Geometry check sheet. Reference: the model listing, model coordinates, mm. A direction names the side the tool comes from. Round coordinates to 2 decimals unless told otherwise and drop trailing zeros. Write each loop counter-clockwise with the first axis right and the second up, starting at its lowest first coordinate (ties: lowest second). Pieces come first, ordered by that corner, then holes. Notation, with made-up numbers: M 68,-28.75 L 73,-28.75 A20 cw 73,-20.75 Z; hole C 77,26.25 d4. An arc over 180 degrees is marked long. Answer in a Markdown table with one row per item. Add a question column.
Autodesk Inventor part; units mm, degrees
ref_plane "YZ Plane" through (0, 0, 0) normal (1, 0, 0) x (0, 1, 0)
ref_plane "XZ Plane" through (0, 0, 0) normal (0, 1, 0) x (-1, 0, 0)
ref_plane "XY Plane" through (0, 0, 0) normal (0, 0, 1) x (1, 0, 0)
sketch "Эскиз1" plane through (0, 0, 0) normal (0, 0, 1) x (1, 0, 0)
  line L0 (115, 5) -> (-115, 5)
  line L1 (-115, 5) -> (-115, -5)
  line L2 (-115, -5) -> (115, -5)
  line L3 (115, -5) -> (115, 5)
  line L4 (115, 5) -> (-115, -5) construction
  line L5 (-115, 5) -> (115, -5) construction
  arc A0 (0, 0) -> (-115, -5) centre (-47.7882, -225.8713) ccw
  arc A1 (115, -5) -> (0, 0) centre (47.7882, -225.8713) ccw
  line L6 (115, 10) -> (-115, 10)
  line L7 (-115, 10) -> (-115, 0)
  line L8 (-115, 0) -> (115, 0)
  line L9 (115, 0) -> (115, 10)
  line L10 (115, 10) -> (-115, 0) construction
  line L11 (-115, 10) -> (115, 0) construction
  arc A2 (0, 5) -> (-115, 0) centre (-47.7882, -220.8713) ccw
  arc A3 (115, 0) -> (0, 5) centre (47.7882, -220.8713) ccw
  line L12 (-115, -5) -> (-95.5764, 5)
  line L13 (115, -5) -> (95.5764, 5)
  line L14 (1.5, 15) -> (-1.5, 15)
  line L15 (-1.5, 15) -> (-1.5, -5)
  line L16 (-1.5, -5) -> (1.5, -5)
  line L17 (1.5, -5) -> (1.5, 15)
  line L18 (1.5, 15) -> (-1.5, -5) construction
  line L19 (-1.5, 15) -> (1.5, -5) construction
  line L20 (-1.5, 5) -> (1.5, 5)
  line L21 (1.5, 5) -> (1.5, 20)
  line L22 (1.5, 20) -> (-1.5, 20)
  line L23 (-1.5, 20) -> (-1.5, 5)
  circle A4 centre (0, 15) radius 1.5
  line L24 (1.5, 20) -> (4.5, 20)
  line L25 (4.5, 20) -> (4.5, 5)
  line L26 (4.5, 5) -> (1.5, 5)
  line L27 (1.5, 5) -> (1.5, 20)
  line L28 (-1.5, 20) -> (-4.5, 20)
  line L29 (-4.5, 20) -> (-4.5, 5)
  line L30 (-4.5, 5) -> (-1.5, 5)
  line L31 (-1.5, 5) -> (-1.5, 20)
  line L32 (-47.7882, 10) -> (-4.5, 10)
  line L33 (4.5, 10) -> (47.7882, 10)
  line L34 (4.5, 13.5) -> (-4.5, 13.5)
  line L35 (-4.5, 13.5) -> (-4.5, 16.5)
  line L36 (-4.5, 16.5) -> (4.5, 16.5)
  line L37 (4.5, 16.5) -> (4.5, 13.5)
  line L38 (4.5, 13.5) -> (-4.5, 16.5) construction
  line L39 (-4.5, 13.5) -> (4.5, 16.5) construction
  line L40 (4.5, 12.5) -> (-4.5, 12.5)
  line L41 (-4.5, 12.5) -> (-4.5, 17.5)
  line L42 (-4.5, 17.5) -> (4.5, 17.5)
  line L43 (4.5, 17.5) -> (4.5, 12.5)
  line L44 (4.5, 12.5) -> (-4.5, 17.5) construction
  line L45 (-4.5, 12.5) -> (4.5, 17.5) construction
  point P0 (1.5, 5.3122)
  point P1 (4.5, 5.9054)
  point P2 (-4.5, 5.9054)
  point P3 (-1.5, 5.3122)
  dimension "d6" = 3
  dimension "d0" = 230
  dimension "d1" = 10
  dimension "d4" = 3
  dimension "d5" = 15
  dimension "d7" = 3
  dimension "d8" = 3
  dimension "d9" = 5
extrude "Выдавливание1" add sketch "Эскиз1" along normal blind 30 contours L13 L8 A1 L0 | L0 L25 A3 | A1 L17 L0 | A3 L25 L6 | L13 A1 L8 | L0 L17 A3 L25 | A1 A0 L15 L0 L17 | L25 A3 L17 L6 | L6 L17 L40 L25 | L40 L17 L34 L25 | A0 L0 L15 | L15 A2 L29 L6 | L6 L29 L40 L15 | L34 L17 L21 L36 L25 | L12 L8 A0 | L0 L29 A2 L15 | L0 A2 L29 | A0 L8 L12 L0 | L29 A2 L6 | L40 L29 L34 L15 | L36 L21 L42 L25 | L34 L29 L36 L23 L15 | L42 L21 L24 L25 | L29 L42 L23 L36 | L42 L29 L28 L23
sketch "Эскиз2" plane through (0, 0, 0) normal (0, 1, 0) x (-1, 0, 0)
  line L0 (115, 0) -> (0, 0)
  line L1 (0, 0) -> (0, 30)
  line L2 (115, 30) -> (0, 30)
  line L3 (115, 0) -> (115, 30)
  line L4 (0, 0) -> (-115, 0)
  line L5 (-115, 0) -> (-115, 30)
  line L6 (0, 30) -> (-115, 30)
  line L7 (0, 0) -> (0, 30)
  line L8 (95.5764, 0) -> (115, 0)
  line L9 (-115, 0) -> (-115, 30)
  line L10 (115, 0) -> (-115, 0)
  line L11 (-115, 0) -> (-115, 15)
  line L12 (-115, 15) -> (115, 15)
  line L13 (115, 15) -> (115, 0)
  line L14 (0, 0) -> (0, 30)
  arc A0 (0, 30) -> (115, 15) centre (102.5177, 367.6359) ccw
  arc A1 (-115, 15) -> (0, 30) centre (-111.4518, 436.1301) ccw
  point P0 (90.0355, 15)
  point P1 (-107.9035, 15)
extrude "Выдавливание2" cut sketch "Эскиз2" along normal mid plane 40 contours L12 A0 L2 L3 | A1 L12 L5 L6
sketch "Эскиз7" plane through (-4.5, 10, 0) normal (-1, 0, 0) x (0, 0, 1)
  line L0 (0, 10) -> (28.6663, 10)
  line L1 (0, 10) -> (5, 10)
  line L2 (5, 10) -> (5, 5)
  line L3 (5, 5) -> (0, 5)
  line L4 (0, 5) -> (0, 10)
  circle A0 centre (5, 5) radius 1.5
  point P0 (0, -10)
  dimension "d68" = 5
  dimension "d69" = 5
  dimension "d70" = 3
extrude "Выдавливание7" cut sketch "Эскиз7" against normal blind 40 contours A0 L3 L2 | L2 L3 A0
properties part number "пиналка_верх"
Item 1: Mould release check, pull along X, two halves, no side actions. Record for faces 5 (the cylindrical face through (-58.63, 4.745, 11.457)), 6 (the flat face through (-0.5, 4.8, 0)), 7 (the cylindrical face through (-38.064, 6.25, 20.716)), 8 (the flat face through (-1.5, 13, 15)): +X half, -X half, draft (parallel to the pull), parting line (faces both ways), or undercut.
Item 2: Scan lines: probe 1 along X at (y, z) = (12, 5); probe 2 along Z at (x, y) = (-2.6, 15); probe 3 along Y at (x, z) = (-3.5, 5). Record each from-to range of solid material in increasing order. Write a range as from..to.
Item 3: Gauge pin test, flat ends, axial feed: pin 1 Ø8 at (y, z) = (16.5, 12) entering from -X; pin 2 Ø1 at (x, y) = (-75, 8) entering from -Z; pin 3 Ø1.5 at (x, z) = (15.5, 17) entering from -Y; pin 4 Ø12 at (x, y) = (-97, 1) entering from +Z. Record the tip position at first contact, or that the pin passes through.
Item 4: Section check C-C, the plane x = -16.5. Record the boundary of the cut face in (y, z).
Item 5: Access from +Z, -Z, +X, -X, +Y, -Y to the whole of each face (thin tool, end or side, straight path). Record for faces 1 (the flat face through (-26, 10, 11)), 2 (the flat face through (4.5, 15, 14)), 3 (the flat face through (-99, 1, 15)), 4 (the flat face through (1.5, 12, 15)).
Item 6: Section check B-B, the plane x = -72.5. Record the boundary of the cut face in (y, z).
Item 7: Section check A-A, the plane z = 13. Record the boundary of the cut face in (x, y).
Result sheet:
| question | item | result |
|---|---|---|
| 1 | face 5 | undercut |
| 1 | face 6 | draft |
| 1 | face 7 | -X half |
| 1 | face 8 | undercut |
| 2 | probe 1 | x = -4.5..-1.5, 1.5..4.5 |
| 2 | probe 2 | z = 0..3.5, 6.5..29.22 |
| 2 | probe 3 | y = 0.71..13.5, 16.5..20 |
| 3 | pin 1 | stops at x = -4.5 |
| 3 | pin 2 | stops at z = 0 |
| 3 | pin 3 | stops at y = 2.62 |
| 3 | pin 4 | stops at z = 15 |
| 4 | outline | M 2.87,0 L 10,0 L 10,25.42 L 2.87,25.42 Z |
| 5 | face 1 | +Z, -Z, -X, +Y |
| 5 | face 2 | +Z, -Z, +X, +Y |
| 5 | face 3 | +Z, -X, +Y, -Y |
| 5 | face 4 | +Z, -Z, +Y |
| 6 | outline | M 3.67,0 L 8.67,0 L 8.67,16.06 L 3.67,16.06 Z |
| 7 | outline | M -115,-5 A230.87 cw 0,0 A230.87 cw 115,-5 L 95.58,5 A230.87 ccw 47.79,10 L 4.5,10 L 4.5,20 L 1.5,20 L 1.5,5 L -1.5,5 L -1.5,20 L -4.5,20 L -4.5,10 L -47.79,10 A230.87 ccw -95.58,5 Z |
